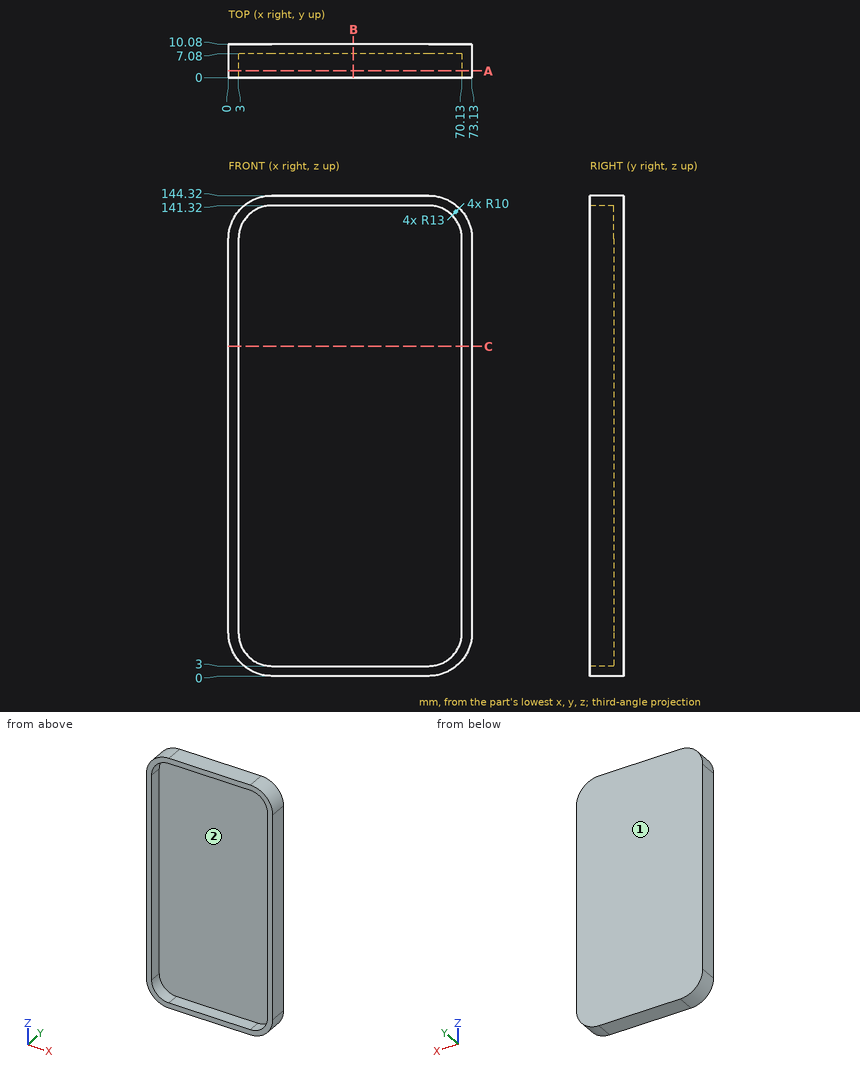
Geometry check sheet. Reference: drawing and pictorial views, mm from the part's lowest x, y, z. Coordinates: 2 decimals unless noted, no trailing zeros. Write each loop counter-clockwise with the first axis right and the second up, starting at its lowest first coordinate (ties: lowest second). Pieces come first, ordered by that corner, then holes. Notation, with made-up numbers: M 80,-6.5 L 118,-6.5 A25 ccw 118,13.5 Z; hole C -16.5,40 d11. An arc over 180 degrees is marked long. Use one line per item in the form item = value.
Item 1: Sectioned sample at B-B, the plane x = 37.5. Record the cut outline in (y, z), and give its area (3 significant figures).
Answer below:
outline = M 0,0 L 10.08,0 L 10.08,144.32 L 0,144.32 L 0,141.32 L 7.08,141.32 L 7.08,3 L 0,3 Z
area = 475 mm^2
Item 2: Sectioned sample at A-A, the plane y = 2. Record the cut outline in (x, z).
Answer below:
outline = M 0,13 A13 ccw 13,0 L 60.13,0 A13 ccw 73.13,13 L 73.13,131.32 A13 ccw 60.13,144.32 L 13,144.32 A13 ccw 0,131.32 Z; hole M 3,13 A10 ccw 13,3 L 60.13,3 A10 ccw 70.13,13 L 70.13,131.32 A10 ccw 60.13,141.32 L 13,141.32 A10 ccw 3,131.32 Z
Item 3: Sectioned sample at C-C, the plane z = 99. Record the cut outline in (x, y).
Answer below:
outline = M 0,0 L 3,0 L 3,7.08 L 70.13,7.08 L 70.13,0 L 73.13,0 L 73.13,10.08 L 0,10.08 Z
Item 4: Release check for a two-part mould opening along Z. For the marked faces 1 and 2 record: pulls with the +Z half, pulls with the -Z half, needs draft (parallel to the pull), parting line crosses it, or undercut.
Answer below:
face_1 = needs draft
face_2 = undercut
Item 5: Material ranges on L1, parallel to X at y = 7, z = 50; L2, parallel to Z at x = 52.5, y = 3.75; L3, parallel to Y at x = 40.5, z = 48.5, recorded low to high. Write a range as from..to.
Answer below:
L1 = 0..3, 70.13..73.13
L2 = 0..3, 141.32..144.32
L3 = 7.08..10.08
